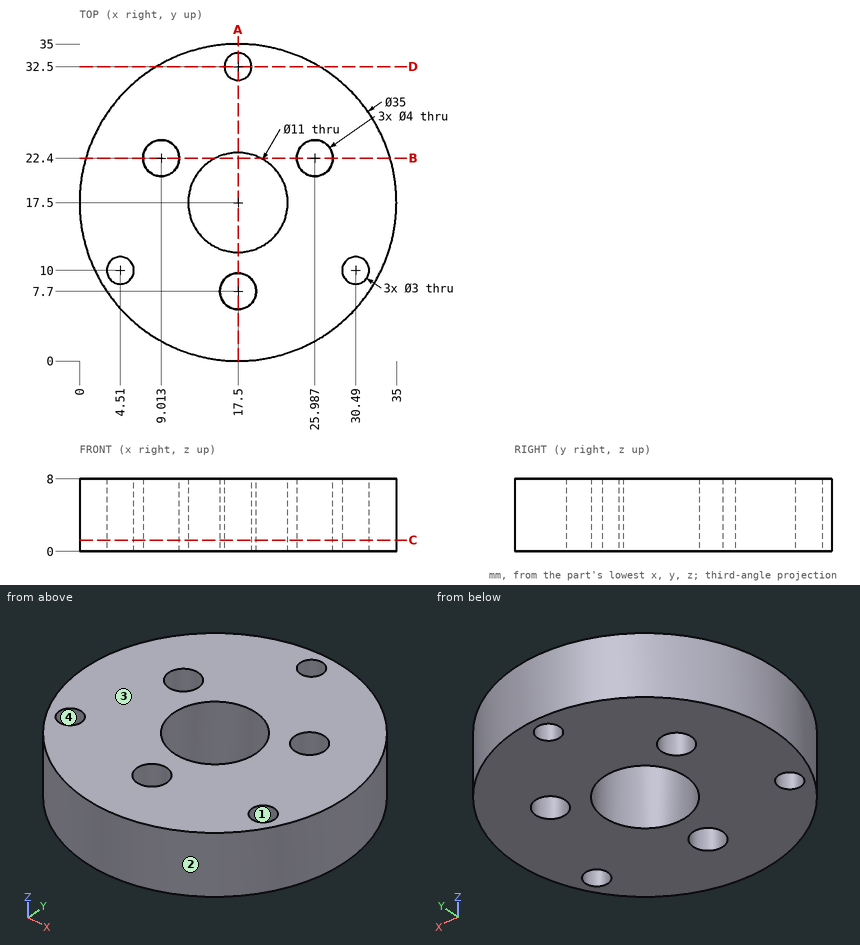
For this review, use the dimensioned drawing (mm, ordinates from the lowest corner) and the shaded views. Round coordinates to 2 decimals unless told otherwise and drop trailing zeros. Order: outer loops, then holes, each group sorted by start corner. A loop starts at its lowest first (then second) coordinate and runs counter-clockwise, first axis right, second up.
1) Draft analysis for pull direction Y (two halves, no side actions). For the marked faces 1, 2, 3 and 4, state which applies: released by +Y, released by -Y, zero draft, split by the parting line, or undercut.
The answers:
face 1: undercut
face 2: split by the parting line
face 3: zero draft
face 4: undercut
2) Consider section C-C (z = 1.25). State the section outline as (x, y) points.
The answers:
outline: circle Ø35 at (17.5, 17.5); hole circle Ø3 at (4.51, 10); hole circle Ø4 at (9.01, 22.4); hole circle Ø11 at (17.5, 17.5); hole circle Ø4 at (17.5, 7.7); hole circle Ø3 at (17.5, 32.5); hole circle Ø4 at (25.99, 22.4); hole circle Ø3 at (30.49, 10)
3) Consider section B-B (y = 22.4). State the section outline as (x, z) points.
The answers:
outline: (0.7, 0) - (7.01, 0) - (7.01, 8) - (0.7, 8) - close; (11.01, 0) - (15, 0) - (15, 8) - (11.01, 8) - close; (20, 0) - (23.99, 0) - (23.99, 8) - (20, 8) - close; (27.99, 0) - (34.3, 0) - (34.3, 8) - (27.99, 8) - close
4) Consider section A-A (x = 17.5). State the section outline as (y, z) points, plus the area to 3 significant figures.
The answers:
outline: (0, 0) - (5.7, 0) - (5.7, 8) - (0, 8) - close; (9.7, 0) - (12, 0) - (12, 8) - (9.7, 8) - close; (23, 0) - (31, 0) - (31, 8) - (23, 8) - close; (34, 0) - (35, 0) - (35, 8) - (34, 8) - close
area: 136 mm2
5) Consider section D-D (y = 32.5). State the section outline as (x, z) points, plus the area to 3 significant figures.
The answers:
outline: (8.49, 0) - (16, 0) - (16, 8) - (8.49, 8) - close; (19, 0) - (26.51, 0) - (26.51, 8) - (19, 8) - close
area: 120 mm2
6) For L1, parallel to Y at x = 17.5, z = 4.25; L2, parallel to X at y = 23.5, z = 3 (1 decimal); L3, parallel to X at y = 21, z = 0.75 (1 decimal), list the stretches that pass through material, from the lowest coordinate up.
The answers:
L1: y = 0 to 5.7, 9.7 to 12, 23 to 31, 34 to 35
L2: x = 1.1 to 7.3, 10.7 to 24.3, 27.7 to 33.9
L3: x = 0.4 to 7.6, 10.4 to 13.3, 21.7 to 24.6, 27.4 to 34.6
7) Clearance check with flat-ended pins moving along their axes: pin 1 Ø2.5 at (x, y) = (30.49, 10) entering from +Z; pin 2 Ø1.5 at (x, z) = (13, 2.5) entering from -Y; pin 3 Ø3 at (y, z) = (7, 4) entering from +X; pin 4 Ø1.5 at (x, z) = (15.5, 3.5) entering from +Y (1 decimal). State where each tip first meets the part, or that it passes through.
The answers:
pin 1: passes through
pin 2: stops at y = 0.41
pin 3: stops at x = 32.51
pin 4: stops at y = 35
